```python
from build123d import *

# Parameters (mm, degrees)
SKETCH1_R           = 10
BOSS_EXTRUDE1_DEPTH = 16
BOSS_EXTRUDE2_DEPTH = 2
SKETCH3_W           = 6
SKETCH3_H           = 14
CUT_EXTRUDE1_DEPTH  = 6.211657


with BuildPart() as part:
    # Sketch1 → Boss-Extrude1 (new body)
    with BuildSketch(Plane(origin=(0, 0, 0), x_dir=(0, 1, 0), z_dir=(0, 0, 1))):
        with BuildLine():
            Line((11.591109915, 3.105828541), (21.591109915, 3.105828541))
            Line((21.591109915, 3.105828541), (21.591109915, -3.105828541))
            Line((21.591109915, -3.105828541), (11.591109915, -3.105828541))
            ThreePointArc((11.591109915, -3.105828541), (-12, 0), (11.591109915, 3.105828541))
        make_face()
        Circle(SKETCH1_R, mode=Mode.SUBTRACT)
    extrude(amount=BOSS_EXTRUDE1_DEPTH)

    # Sketch2 → Boss-Extrude2 (add)
    with BuildSketch(Plane(origin=(0, 0, 0), x_dir=(1, 0, 0), z_dir=(0, 0, -1))):
        with BuildLine():
            Line((-3.105828541, -21.591109915), (3.105828541, -21.591109915))
            Line((3.105828541, -21.591109915), (3.105828541, -11.591109915))
            ThreePointArc((3.105828541, -11.591109915), (0, 12), (-3.105828541, -11.591109915))
            Line((-3.105828541, -11.591109915), (-3.105828541, -21.591109915))
        make_face()
    extrude(amount=BOSS_EXTRUDE2_DEPTH)

    # Sketch3 → Cut-Extrude1 (cut)
    with BuildSketch(Plane.YZ.offset(3.105828541)):
        with Locations((16.591109915, 7)):
            Rectangle(SKETCH3_W, SKETCH3_H)
    extrude(amount=-CUT_EXTRUDE1_DEPTH, mode=Mode.SUBTRACT)


solid = part.part
```
Check sheet for the modelled part. Datum: model origin and axes. Units: mm. A direction names the side the tool comes from. Coordinates: 2 decimals unless noted, no trailing zeros. Loops run counter-clockwise (first coordinate to the right, second up) from the corner with the lowest first, then second, coordinate; pieces in that order, holes last. Notation, with made-up numbers: M -7,-3.5 L 46,-3.5 A27 ccw 46,25.5 Z; hole C 64.5,-37.75 d5. An arc over 180 degrees is marked long. Answer as a JSON object with one key per item and string values.
1. Access from +Z, -Z, +X, -X, +Y, -Y to the whole of each face (thin tool, end or side, straight path). Record for faces 1 (the flat face through (3.106, 13, 7)), 2 (the flat face through (0, 0, 0)), 3 (the flat face through (0, 17, 14)), 4 (the cylindrical face through (0, -12, 7)), 5 (the flat face through (0, 1, -2)).
Outcome:
{"face 1": "+Z, -Z, +X, +Y", "face 2": "+Z", "face 3": "+X, -X", "face 4": "+Z, -Z", "face 5": "-Z, +X, -X, +Y, -Y"}
2. Sectioned sample at D-D on x = -8. Record the cut outline in (y, z).
Outcome:
{"outline": "M -8.94,-2 L 8.94,-2 L 8.94,16 L 6,16 L 6,0 L -6,0 L -6,16 L -8.94,16 Z"}
3. Release check for a two-part mould opening along X. For faces 6 (the cylindrical face through (9.76, -2.17, 7.89)), 7 (the flat face through (-3.106, 20, 7)), 8 (the flat face through (0, 21.591, 7)) record: pulls with the +X half, pulls with the -X half, needs draft (parallel to the pull), parting line crosses it, or undercut.
Outcome:
{"face 6": "undercut", "face 7": "pulls with the -X half", "face 8": "needs draft"}
4. Sectioned sample at A-A on z = 8. Record the cut outline in (x, y), and give its area (3 significant figures).
Outcome:
{"outline": "M -3.11,11.59 A12 ccw long 3.11,11.59 L 3.11,13.59 L -3.11,13.59 Z; M -3.11,19.59 L 3.11,19.59 L 3.11,21.59 L -3.11,21.59 Z; hole C 0,0 d20", "area": "161 mm²"}
5. Sectioned sample at B-B on x = -1.75. Record the cut outline in (y, z), and give its area (3 significant figures).
Outcome:
{"outline": "M -11.87,-2 L 21.59,-2 L 21.59,16 L 9.85,16 L 9.85,0 L -9.85,0 L -9.85,16 L -11.87,16 Z; hole M 13.59,0 L 19.59,0 L 19.59,14 L 13.59,14 Z", "area": "203 mm²"}
6. Sectioned sample at C-C on y = 0. Record the cut outline in (x, z), and give its area (3 significant figures).
Outcome:
{"outline": "M -12,-2 L 12,-2 L 12,16 L 10,16 L 10,0 L -10,0 L -10,16 L -12,16 Z", "area": "112 mm²"}
7. Scan lines: L1, parallel to Y at x = -0.25, z = 13; L2, parallel to X at y = 0, z = 8.25; L3, parallel to Z at x = 2.5, y = 14.5. Record each from-to range of solid material in increasing order. Write a range as from..to.
Outcome:
{"L1": "-12..-10, 10..13.59, 19.59..21.59", "L2": "-12..-10, 10..12", "L3": "-2..0, 14..16"}
8. Depth check by flat-ended pin: P1, Ø10, axis at x = 1, y = 4, coming from the +Z side; P2, Ø2, axis at x = 9, z = 14, coming from the -Y side; P3, Ø3, axis at y = 18.5, z = 7.5, coming from the +X side; P4, Ø3, axis at y = 17, z = 6, coming from the -X side. Enter the tip coordinate at first touch or a pass-through.
Outcome:
{"P1": "z = 0", "P2": "y = -8.94", "P3": "x = 3.11", "P4": "through"}
